Work out the finished part from the listing and answer in its coordinate system (mm). A direction names the side the tool comes from. Give positions to 0.01 mm unless a question says otherwise; leave off trailing zeros. Order: outer loops, then holes, each group sorted by start corner. A loop starts at its lowest first (then second) coordinate and runs counter-clockwise, first axis right, second up. Notation, with made-up numbers: (46.25, 48.5) -> (62.25, 48.5) arc R24 ccw to (62.25, 78.5) -> close; hole circle Ø8 at (24, 19). An arc over 180 degrees is marked (long way). Use a Markdown table: item, result. Add a question column.
```python
from build123d import *

# Parameters (mm, degrees)
F0_R     = 1.6
F0_W     = 92.3
F0_H     = 6.35
F0_W_2   = 6.35
F0_H_2   = 92.3
F1_DEPTH = 58.42
F2_W     = 48.1660993379
F2_H     = 92.3
F3_DEPTH = 25.4
F4_W     = 92.3
F4_H     = 48.2718696427
F5_DEPTH = 25.4
F6_W     = 47.9031776619
F6_H     = 92.3
F7_DEPTH = 25.4
F8_W     = 92.3
F8_H     = 47.8445788455
F9_DEPTH = 25.4


with BuildPart() as f1:
    # F0 (on Front) → F1 (new body)
    with BuildSketch(Plane.XZ):
        Polygon((-98.65, 105), (-98.65, 111.35), (-111.35, 111.35), (-111.35, 98.65), (-105, 98.65), (-98.65, 98.65), align=None)
        with Locations((-105, 105)):
            Circle(F0_R, mode=Mode.SUBTRACT)
        with Locations((-52.5, 101.825)):
            Rectangle(F0_W, F0_H)
        with Locations((-101.825, 52.5)):
            Rectangle(F0_W_2, F0_H_2)
        Polygon((-6.35, 111.35), (-6.35, 105), (-6.35, 98.65), (0, 98.65), (6.35, 98.65), (6.35, 111.35), align=None)
        with Locations((0, 105)):
            Circle(F0_R, mode=Mode.SUBTRACT)
        Polygon((-98.65, 0), (-98.65, 6.35), (-105, 6.35), (-111.35, 6.35), (-111.35, -6.35), (-98.65, -6.35), align=None)
        with Locations((-105, 0)):
            Circle(F0_R, mode=Mode.SUBTRACT)
        with Locations((-52.5, 3.175)):
            Rectangle(F0_W, F0_H)
        with Locations((-3.175, 52.5)):
            Rectangle(F0_W_2, F0_H_2)
        with BuildLine():
            Line((0, 6.35), (-6.35, 6.35))
            Line((-6.35, 6.35), (-6.35, 0))
            Line((-6.35, 0), (-1.6, 0))
            ThreePointArc((-1.6, 0), (-1.1313708499, 1.1313708499), (0, 1.6))
            Line((0, 1.6), (0, 6.35))
        make_face()
        with BuildLine():
            Line((-1.6, 0), (-6.35, 0))
            Line((-6.35, 0), (-6.35, -6.35))
            Line((-6.35, -6.35), (6.35, -6.35))
            Line((6.35, -6.35), (6.35, 6.35))
            Line((6.35, 6.35), (0, 6.35))
            Line((0, 6.35), (0, 1.6))
            ThreePointArc((0, 1.6), (1.1313708499, 1.1313708499), (1.6, 0))
            ThreePointArc((1.6, 0), (0, -1.6), (-1.6, 0))
        make_face()
    extrude(amount=F1_DEPTH)

    # F2 (on face) → F3 (cut)
    with BuildSketch(Plane(origin=(-105, 0, 0), x_dir=(0, -1, 0), z_dir=(-1, 0, 0))):
        with Locations((34.336950331, 52.5)):
            Rectangle(F2_W, F2_H)
    extrude(amount=-F3_DEPTH, mode=Mode.SUBTRACT)

    # F4 (on face) → F5 (cut)
    with BuildSketch(Plane(origin=(0, 0, 0), x_dir=(1, 0, 0), z_dir=(0, 0, -1))):
        with Locations((-52.5, 34.2840651786)):
            Rectangle(F4_W, F4_H)
    extrude(amount=-F5_DEPTH, mode=Mode.SUBTRACT)

    # F6 (on face) → F7 (cut)
    with BuildSketch(Plane.YZ):
        with Locations((-34.4684111691, 52.5)):
            Rectangle(F6_W, F6_H)
    extrude(amount=-F7_DEPTH, mode=Mode.SUBTRACT)

    # F8 (on face) → F9 (cut)
    with BuildSketch(Plane.XY.offset(105)):
        with Locations((-52.5, -34.4977105772)):
            Rectangle(F8_W, F8_H)
    extrude(amount=-F9_DEPTH, mode=Mode.SUBTRACT)


solid = f1.part
```
1) Flat-ended cylindrical pins translate along their axes: pin 1 (11 mm diameter, centred on x = -70.5, y = -4, fed in from -Z); pin 2 (2.5 mm diameter, centred on x = 0, z = 105, fed in from -Y); pin 3 (7 mm diameter, centred on x = -3, z = 48.5, fed in from -Y); pin 4 (5.5 mm diameter, centred on x = -54, y = -3.5, fed in from +Z). Find the tip coordinate at first contact, or state that the pin passes through.
2) Determine the mould class of faces 4 (the cylindrical face through (-106.6, -28.8, 0.07)), 5 (the flat face through (-98.65, -10, 34)), 6 (the flat face through (0, -5, 52)), 7 (the flat face through (-2, -58.42, 107)) for opening direction X: released by +X, released by -X, zero draft, split by the parting line, or undercut.
3) The part is cut by section A-A, the plane y = -52. Determine the outline of the cut face in (x, z), then the cut area to 3 significant figures.
4) The part is cut by section B-B, the plane x = -38.5. Determine the outline of the cut face in (y, z), then the cut area to 3 significant figures.
5) The part is cut by section C-C, the plane y = -6. Determine the outline of the cut face in (x, z), then the cut area to 3 significant figures.
6) Straight lines are drawn through the part: line 1 (Z direction, x = -105, y = -19); line 2 (X direction, y = -53, z = 105); line 3 (X direction, y = -3.5, z = 96.5). For each, find the intervals that lie inside material, in ascending order.
7) The part is cut by section D-D, the plane z = 86.5. Determine the outline of the cut face in (x, y), then the cut area to 3 significant figures.
8) Which of the six approach directions +Z, -Z, +X, -X, +Y, -Y give full straight-line access (tool end or side, diameter ignored) to faces 1 (the flat face through (-105, -5, 52)), 2 (the flat face through (-53, -10.148, 3)), 3 (the flat face through (-53, -5, 0))?
A:
| question | item | result |
|---|---|---|
| 1 | pin 1 | z = 0 |
| 1 | pin 2 | through |
| 1 | pin 3 | y = -10.52 |
| 1 | pin 4 | z = 105 |
| 2 | face 4 | undercut |
| 2 | face 5 | undercut |
| 2 | face 6 | released by +X |
| 2 | face 7 | zero draft |
| 3 | outline | (-111.35, -6.35) -> (-98.65, -6.35) -> (-98.65, 6.35) -> (-111.35, 6.35) -> close; (-111.35, 98.65) -> (-98.65, 98.65) -> (-98.65, 111.35) -> (-111.35, 111.35) -> close; (-6.35, -6.35) -> (6.35, -6.35) -> (6.35, 6.35) -> (-6.35, 6.35) -> close; (-6.35, 98.65) -> (6.35, 98.65) -> (6.35, 111.35) -> (-6.35, 111.35) -> close; hole circle Ø3.2 at (-105, 0); hole circle Ø3.2 at (-105, 105); hole circle Ø3.2 at (0, 0); hole circle Ø3.2 at (0, 105) |
| 3 | area | 613 mm^2 |
| 4 | outline | (-10.58, 98.65) -> (0, 98.65) -> (0, 105) -> (-10.58, 105) -> close; (-10.15, 0) -> (0, 0) -> (0, 6.35) -> (-10.15, 6.35) -> close |
| 4 | area | 132 mm^2 |
| 5 | outline | (-111.35, -6.35) -> (-98.65, -6.35) -> (-98.65, 0) -> (-6.35, 0) -> (-6.35, -6.35) -> (6.35, -6.35) -> (6.35, 6.35) -> (0, 6.35) -> (0, 98.65) -> (6.35, 98.65) -> (6.35, 111.35) -> (-6.35, 111.35) -> (-6.35, 105) -> (-98.65, 105) -> (-98.65, 111.35) -> (-111.35, 111.35) -> (-111.35, 98.65) -> (-105, 98.65) -> (-105, 6.35) -> (-111.35, 6.35) -> close; hole circle Ø3.2 at (-105, 0); hole circle Ø3.2 at (-105, 105); hole (-98.65, 6.35) -> (-6.35, 6.35) -> (-6.35, 98.65) -> (-98.65, 98.65) -> close; hole circle Ø3.2 at (0, 0); hole circle Ø3.2 at (0, 105) |
| 5 | area | 2,960 mm^2 |
| 6 | line 1 | -6.35 to -1.6, 1.6 to 6.35, 98.65 to 103.4, 106.6 to 111.35 |
| 6 | line 2 | -111.35 to -106.6, -103.4 to -98.65, -6.35 to -1.6, 1.6 to 6.35 |
| 6 | line 3 | -105 to -98.65, -6.35 to 0 |
| 7 | outline | (-105, -10.25) -> (-98.65, -10.25) -> (-98.65, 0) -> (-105, 0) -> close; (-6.35, -10.52) -> (0, -10.52) -> (0, 0) -> (-6.35, 0) -> close |
| 7 | area | 132 mm^2 |
| 8 | face 1 | -X, +Y, -Y |
| 8 | face 2 | -Z, -Y |
| 8 | face 3 | -Z, +Y, -Y |
